```python
from build123d import *

# Parameters (mm, degrees)
SKETCH1_W                    = 94.361
SKETCH1_H                    = 38.1
BASE_FLANGE1_DEPTH           = 2.286
EDGE_FLANGE1_STRIP_W         = 10.6172
EDGE_FLANGE1_STRIP_H         = 2.286
EDGE_FLANGE1_STRIP_CUT_DEPTH = 38.1
EDGE_FLANGE1_DEPTH           = 38.1
EDGE_FLANGE2_STRIP_W         = 10.6172
EDGE_FLANGE2_STRIP_H         = 2.286
EDGE_FLANGE2_STRIP_CUT_DEPTH = 38.1
EDGE_FLANGE2_DEPTH           = 38.1


# Sheet-metal steps are written as plain solids
with BuildPart() as part:
    # Sketch1 → Base-Flange1 (new body)
    with BuildSketch(Plane(origin=(0, 0, 0), x_dir=(1, 0, 0), z_dir=(0, 1, 0))):
        Rectangle(SKETCH1_W, SKETCH1_H)
    extrude(amount=-BASE_FLANGE1_DEPTH)

    # Edge-Flange1 strip (across the edge) → Edge-Flange1 strip cut (cut)
    with BuildSketch(Plane(origin=(47.1805, 0, 19.05), x_dir=(-1, 0, 0), z_dir=(0, 0, -1))):
        with Locations((-2.286, -1.143)):
            Rectangle(EDGE_FLANGE1_STRIP_W, EDGE_FLANGE1_STRIP_H)
    extrude(amount=EDGE_FLANGE1_STRIP_CUT_DEPTH, mode=Mode.SUBTRACT)

    # Edge-Flange1 section (across the edge) → Edge-Flange1 (add)
    with BuildSketch(Plane(origin=(47.1805, 0, 19.05), x_dir=(-1, 0, 0), z_dir=(0, 0, -1))):
        with BuildLine():
            Line((0, 0.7366), (0, 37.4015))
            Line((0, 37.4015), (2.286, 37.4015))
            Line((2.286, 37.4015), (2.286, 0.7366))
            ThreePointArc((2.286, 0.7366), (2.501745145, 0.215745145), (3.0226, 0))
            Line((3.0226, 0), (3.0226, -2.286))
            ThreePointArc((3.0226, -2.286), (0.885299043, -1.400700957), (0, 0.7366))
        make_face()
    extrude(amount=EDGE_FLANGE1_DEPTH)

    # Edge-Flange2 strip (across the edge) → Edge-Flange2 strip cut (cut)
    with BuildSketch(Plane(origin=(-47.1805, 0, -19.05), x_dir=(1, 0, 0), z_dir=(0, 0, 1))):
        with Locations((-2.286, -1.143)):
            Rectangle(EDGE_FLANGE2_STRIP_W, EDGE_FLANGE2_STRIP_H)
    extrude(amount=EDGE_FLANGE2_STRIP_CUT_DEPTH, mode=Mode.SUBTRACT)

    # Edge-Flange2 section (across the edge) → Edge-Flange2 (add)
    with BuildSketch(Plane(origin=(-47.1805, 0, -19.05), x_dir=(1, 0, 0), z_dir=(0, 0, 1))):
        with BuildLine():
            Line((0, 0.7366), (0, 70.739))
            Line((0, 70.739), (2.286, 70.739))
            Line((2.286, 70.739), (2.286, 0.7366))
            ThreePointArc((2.286, 0.7366), (2.501745145, 0.215745145), (3.0226, 0))
            Line((3.0226, 0), (3.0226, -2.286))
            ThreePointArc((3.0226, -2.286), (0.885299043, -1.400700957), (0, 0.7366))
        make_face()
    extrude(amount=EDGE_FLANGE2_DEPTH)


solid = part.part
```
CAD build for the part. Positions are in the model's coordinates, mm. A direction names the side the tool comes from. Round coordinates to 2 decimals unless told otherwise and drop trailing zeros. Order: outer loops, then holes, each group sorted by start corner. A loop starts at its lowest first (then second) coordinate and runs counter-clockwise, first axis right, second up.
Item 1: Probe line 1 along X through (y, z) = (3, 11.5); line 2 along X through (y, z) = (49.5, -10.5); line 3 along Y through (x, z) = (-33.5, -7). List the from-to ranges inside material, lowest first.
Item 2: Mould opens along X. For faces 4 (the face through (-1, 0, 0)), 5 (the face through (-7, -1, -19.05)), 6 (the face through (-46.272, -1.424, -0.267)) say: pulls with the +X half, pulls with the -X half, needs draft (parallel to the pull), parting line crosses it, or undercut.
Item 3: Saw through at D-D on y = 40.5. Write the cut outline in (x, z), then the cut area to 3 significant figures.
Item 4: Saw through at B-B on z = 7.5. Write the cut outline in (x, y), then the cut area to 3 significant figures.
Item 5: Pin check, flat tips, straight feed: pin 1 (19 mm diameter, centred on x = -7.5, z = 2, fed in from +Y); pin 2 (1.1 mm diameter, centred on x = 46.5, z = -0.5, fed in from +Y); pin 3 (12 mm diameter, centred on x = 36.5, y = 13.5, fed in from -Z); pin 4 (12 mm diameter, centred on y = 45, z = 15, fed in from +X). Stop position of each tip, or through.
Item 6: Tool access for faces 1 (the face through (44.894, 19, 0)), 2 (the face through (47.18, 19, 0)), 3 (the face through (46, 37.402, 0)): list every direction of +Z, -Z, +X, -X, +Y, -Y with a clear straight run to the whole face (end or side of a thin tool).
Item 7: Saw through at C-C on x = 24. Write the cut outline in (y, z), then the cut area to 3 significant figures.
Item 8: Saw through at A-A on y = 5.5. Write the cut outline in (x, z), then the cut area to 3 significant figures.
Reported:
1. line 1: x = -47.18 to -44.89, 44.89 to 47.18
1. line 2: x = -47.18 to -44.89
1. line 3: y = -2.29 to 0
2. face 4: undercut
2. face 5: needs draft
2. face 6: pulls with the -X half
3. outline: (-47.18, -19.05) - (-44.89, -19.05) - (-44.89, 19.05) - (-47.18, 19.05) - close
3. area: 87.1 mm2
4. outline: (-47.18, 0.74) arc R3.02 ccw to (-44.16, -2.29) - (44.16, -2.29) arc R3.02 ccw to (47.18, 0.74) - (47.18, 37.4) - (44.89, 37.4) - (44.89, 0.74) arc R0.74 cw to (44.16, 0) - (-44.16, 0) arc R0.74 cw to (-44.89, 0.74) - (-44.89, 70.74) - (-47.18, 70.74) - close
4. area: 459 mm2
5. pin 1: stops at y = 0
5. pin 2: stops at y = 37.4
5. pin 3: passes through
5. pin 4: stops at x = -44.89
6. face 1: +Z, -Z, +Y
6. face 2: +Z, -Z, +X, +Y, -Y
6. face 3: +Z, -Z, +X, +Y
7. outline: (-2.29, -19.05) - (0, -19.05) - (0, 19.05) - (-2.29, 19.05) - close
7. area: 87.1 mm2
8. outline: (-47.18, -19.05) - (-44.89, -19.05) - (-44.89, 19.05) - (-47.18, 19.05) - close; (44.89, -19.05) - (47.18, -19.05) - (47.18, 19.05) - (44.89, 19.05) - close
8. area: 174 mm2
